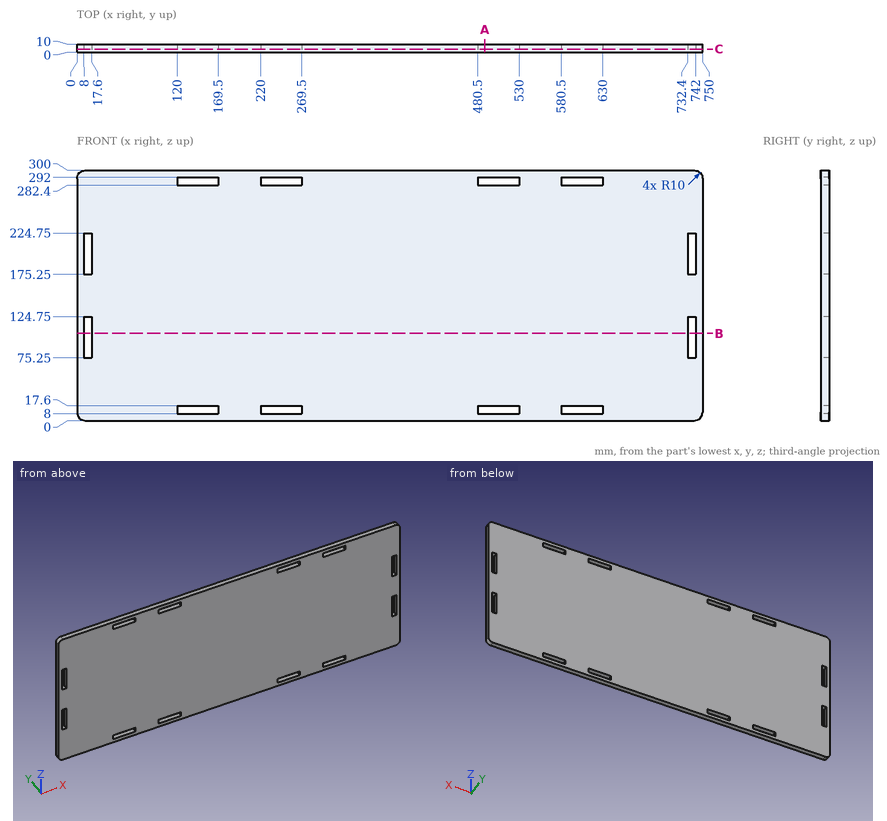
Drawing for the job (mm, zero at the part's lowest x, y, z). Give positions to 0.01 mm unless a question says otherwise; leave off trailing zeros. Loops run counter-clockwise (first coordinate to the right, second up) from the corner with the lowest first, then second, coordinate; pieces in that order, holes last.
Item 1: Drill centre lines: line 1 along X through (y, z) = (6.5, 201.5); line 2 along Z through (x, y) = (225, 7.25); line 3 along X through (y, z) = (2, 14). Where is each one in solid material? Low to high.
Check values:
line 1: x = 0 to 8, 17.6 to 732.4, 742 to 750
line 2: z = 0 to 8, 17.6 to 282.4, 292 to 300
line 3: x = 0 to 120, 169.5 to 220, 269.5 to 480.5, 530 to 580.5, 630 to 750
Item 2: Slice it at A-A (x = 489). Write the cut outline in (y, z).
Check values:
outline: (0, 0) - (10, 0) - (10, 8) - (0, 8) - close; (0, 17.6) - (10, 17.6) - (10, 282.4) - (0, 282.4) - close; (0, 292) - (10, 292) - (10, 300) - (0, 300) - close
Item 3: Slice it at B-B (z = 104.5). Write the cut outline in (x, y), plus the area to 3 significant figures.
Check values:
outline: (0, 0) - (8, 0) - (8, 10) - (0, 10) - close; (17.6, 0) - (732.4, 0) - (732.4, 10) - (17.6, 10) - close; (742, 0) - (750, 0) - (750, 10) - (742, 10) - close
area: 7,310 mm2
Item 4: Slice it at C-C (y = 4). Give the number of separate pieces and of enclosed holes in the cut face, plus the area to 3 significant figures.
Check values:
separate pieces: 1
enclosed holes: 12
area: 219,000 mm2
